```python
from build123d import *

# Parameters (mm, degrees)
F0_W     = 0.8
F0_H     = 32
F1_DEPTH = 6.3
F3_R     = 2.5
F4_DEPTH = 11
F5_R     = 2
F6_F1_R  = 0.4
F6_F2_R  = 0.4
F7_R     = 1


# Not quite as in the source:
# - a feature names something its author has since deleted; it is built from what else it names


with BuildPart() as f1:
    # F0 (on Front) → F1 (new body, symmetric)
    with BuildSketch(Plane.XZ):
        with BuildLine():
            Line((34, 24), (-34, 24))
            ThreePointArc((-34, 24), (-38.2426406871, 22.2426406871), (-40, 18))
            Line((-40, 18), (-40, -18))
            ThreePointArc((-40, -18), (-38.2426406871, -22.2426406871), (-34, -24))
            Line((-34, -24), (34, -24))
            ThreePointArc((34, -24), (38.2426406871, -22.2426406871), (40, -18))
            Line((40, -18), (40, 18))
            ThreePointArc((40, 18), (38.2426406871, 22.2426406871), (34, 24))
        make_face()
        with Locations((-38.8, 0)):
            Rectangle(F0_W, F0_H, mode=Mode.SUBTRACT)
        with BuildLine():
            ThreePointArc((-36, 11), (-33.3639610307, 17.3639610307), (-27, 20))
            Line((-27, 20), (34, 20))
            ThreePointArc((34, 20), (35.4142135624, 19.4142135624), (36, 18))
            Line((36, 18), (36, -11))
            ThreePointArc((36, -11), (33.3639610307, -17.3639610307), (27, -20))
            Line((27, -20), (-34, -20))
            ThreePointArc((-34, -20), (-35.4142135624, -19.4142135624), (-36, -18))
            Line((-36, -18), (-36, 11))
        make_face(mode=Mode.SUBTRACT)
        with Locations((38.8, 0)):
            Rectangle(F0_W, F0_H, mode=Mode.SUBTRACT)
    extrude(amount=F1_DEPTH, both=True)

    # F3 (on offset) → F4 (cut)
    with BuildSketch(Plane.XZ.offset(5.5)):
        with Locations((-34.9874263129, 20.2)):
            Circle(F3_R)
        with Locations((34.9874263129, -20.2)):
            Circle(F3_R)
    extrude(amount=-F4_DEPTH, mode=Mode.SUBTRACT)

    # F5
    f5_edges = [f1.edges().sort_by_distance(p)[0] for p in [
        (-38.4, 6.3, 0),
        (38.4, 6.3, 0),
    ]]
    fillet(f5_edges, radius=F5_R)

    # F6: fillet of radius 0.4 on 8 edges, made by hand

    # F6_f1
    f6_f1_edges = [f1.edges().sort_by_distance(p)[0] for p in [
        (-39.2, 0, 16),
        (-39.2, 0, -16),
        (39.2, 0, -16),
        (39.2, 0, 16),
    ]]
    fillet(f6_f1_edges, radius=F6_F1_R)

    # F6_f2
    f6_f2_edges = [f1.edges().sort_by_distance(p)[0] for p in [
        (38.6, 6.3, 16),
        (-38.6, 6.3, 16),
        (-39.2, 6.3, 0),
        (39.2, 6.3, 0),
        (-37.4, 6.3, 16),
        (37.4, 6.3, 16),
        (39.0828427125, 6.3, 15.8828427125),
        (39.0828427125, 6.3, -15.8828427125),
        (-39.0828427125, 6.3, -15.8828427125),
        (-39.0828427125, 6.3, 15.8828427125),
    ]]
    fillet(f6_f2_edges, radius=F6_F2_R)

    # F7
    f7_edges = [f1.edges().sort_by_distance(p)[0] for p in [
        (38.4, -6.3, 0),
        (39.2, -6.3, 0),
        (-38.4, -6.3, 0),
        (-39.2, -6.3, 0),
        (38.6, -6.3, -16),
        (38.6, -6.3, 16),
        (-38.6, -6.3, -16),
        (-38.6, -6.3, 16),
    ]]
    fillet(f7_edges, radius=F7_R)


solid = f1.part
```
The model under review builds one solid part; all positions refer to its coordinate system, in mm. A direction names the side the tool comes from. Give positions to 0.01 mm unless a question says otherwise; leave off trailing zeros. Write each loop counter-clockwise with the first axis right and the second up, starting at its lowest first coordinate (ties: lowest second). Pieces come first, ordered by that corner, then holes.
(1) Consider section B-B, the plane y = -3.75. Give the number of separate pieces and of enclosed holes in the cut face, and give its area (3 significant figures).
(2) Consider section C-C, the plane z = -19. Give the boundary of the cut face in (x, y), and give its area (3 significant figures).
(3) Consider section A-A, the plane x = -12. Give the boundary of the cut face in (y, z).
(4) Tool access review of faces 4 (the cylindrical face through (37.297, -0.077, -21.158)), 5 (the cylindrical face through (37.8, 5.73, 0.23)), 6 (the cylindrical face through (35.4, -0.09, 19.43)), 7 (the flat face through (-40, 0, 0)): name each direction out of +Z, -Z, +X, -X, +Y, -Y from which nothing blocks a thin tool from reaching the whole face with its end or side.
(5) For P1, Ø1.3, axis at x = -38.5, y = 1.5, coming from the +Z side; P2, Ø0.6, axis at x = 38, y = -2, coming from the -Z side; P3, Ø1.3, axis at x = 38, y = -1.5, coming from the +Z side, all flat-tipped, find the tip position at first contact; note any pin that passes through.
(6) The part is to be moulded in two halves that separate along Y. For faces 1 (the flat face through (0, -6.3, -21)), 2 (the flat face through (40, 0, 0)), 3 (the flat face through (-35, 5.5, 20)), say which applies: released by +Y, released by -Y, zero draft, split by the parting line, or undercut.
(7) To check wall thickness, follow L1, parallel to X at y = -3.5, z = -5; L2, parallel to X at y = 5.5, z = -14.5; L3, parallel to Z at x = 0.5, y = 0. State the ranges of each line that lie inside material, in increasing order.
Returned:
1. separate pieces: 1
1. enclosed holes: 5
1. area: 875 mm2
2. outline: (-39.92, -6.3) - (-35.73, -6.3) - (-35.73, 6.3) - (-39.92, 6.3) - close; (31.12, -6.3) - (39.92, -6.3) - (39.92, 6.3) - (31.12, 6.3) - close; hole (32.79, -5.5) - (37.18, -5.5) - (37.18, 5.5) - (32.79, 5.5) - close
2. area: 115 mm2
3. outline: (-6.3, -24) - (6.3, -24) - (6.3, -20) - (-6.3, -20) - close; (-6.3, 20) - (6.3, 20) - (6.3, 24) - (-6.3, 24) - close
4. face 4: none
4. face 5: +Y
4. face 6: +Y, -Y
4. face 7: +Z, -Z, -X, +Y, -Y
5. P1: stops at z = 22.6
5. P2: stops at z = -22.72
5. P3: stops at z = 22.98
6. face 1: released by -Y
6. face 2: zero draft
6. face 3: undercut
7. L1: x = -40 to -39.2, -38.4 to -36, 36 to 38.4, 39.2 to 40
7. L2: x = -40 to -39.2, -38 to -36, 35.29 to 38, 39.2 to 40
7. L3: z = -24 to -20, 20 to 24
